The model under review builds one solid part; all positions refer to its coordinate system, in mm. A direction names the side the tool comes from. Coordinates: 2 decimals unless noted, no trailing zeros. Write each loop counter-clockwise with the first axis right and the second up, starting at its lowest first coordinate (ties: lowest second). Pieces come first, ordered by that corner, then holes.
```python
from build123d import *

# Parameters (mm, degrees)
ESBO_O1_W                                            = 105
ESBO_O1_H                                            = 50
RESSALTO_EXTRUS_O1_DEPTH                             = 6.35
FURO_DE_DI_METRO_2_5_2_5_1_D                         = 2.5
FURO_DE_DI_METRO_2_5_2_5_1_DEPTH                     = 6.35
REBAIXO_PARA_PARAFUSO_DE_M_QUINA_DE_CABE_D           = 2.2
REBAIXO_PARA_PARAFUSO_DE_M_QUINA_DE_CABE_DEPTH       = 6.35
REBAIXO_PARA_PARAFUSO_DE_M_QUINA_DE_CABE_CBORE_D     = 4.4
REBAIXO_PARA_PARAFUSO_DE_M_QUINA_DE_CABE_CBORE_DEPTH = 2.25
REBAIXO_PARA_PARAFUSO_DE_M_QUINA_DE_2_D              = 4.3
REBAIXO_PARA_PARAFUSO_DE_M_QUINA_DE_2_CBORE_D        = 8
REBAIXO_PARA_PARAFUSO_DE_M_QUINA_DE_2_CBORE_DEPTH    = 4.25
REBAIXO_PARA_PARAFUSO_DE_M_QUINA_DE_3_D              = 4.3
REBAIXO_PARA_PARAFUSO_DE_M_QUINA_DE_3_DEPTH          = 6.35
REBAIXO_PARA_PARAFUSO_DE_M_QUINA_DE_3_CBORE_D        = 8
REBAIXO_PARA_PARAFUSO_DE_M_QUINA_DE_3_CBORE_DEPTH    = 4.25
FILETE1_R                                            = 3
ESBO_O11_R                                           = 4
RESSALTO_EXTRUS_O2_DEPTH                             = 6.35


with BuildPart() as part:
    # Esboço1 → Ressalto-extrusão1 (new body)
    with BuildSketch(Plane.XY.offset(6.35)):
        with Locations((52.5, 12)):
            Rectangle(ESBO_O1_W, ESBO_O1_H)
    extrude(amount=-RESSALTO_EXTRUS_O1_DEPTH)

    # Furo de diâmetro Ø2.5 (2.5)1
    with Locations(Plane(origin=(0, 0, 0), x_dir=(-1, 0, 0), z_dir=(0, 0, -1))):
        with Locations((-95.5, 17), (-95.5, 7)):
            Hole(FURO_DE_DI_METRO_2_5_2_5_1_D / 2, depth=FURO_DE_DI_METRO_2_5_2_5_1_DEPTH)

    # Rebaixo para parafuso de m_quina de cabe
    with Locations(Plane.XY.offset(6.35)):
        with Locations((45.856, 22), (45.856, 2), (45.856, 12)):
            CounterBoreHole(REBAIXO_PARA_PARAFUSO_DE_M_QUINA_DE_CABE_D / 2, REBAIXO_PARA_PARAFUSO_DE_M_QUINA_DE_CABE_CBORE_D / 2, REBAIXO_PARA_PARAFUSO_DE_M_QUINA_DE_CABE_CBORE_DEPTH, depth=REBAIXO_PARA_PARAFUSO_DE_M_QUINA_DE_CABE_DEPTH)

    # Rebaixo para parafuso de m_quina de  2 (through all)
    with Locations(Plane(origin=(0, 0, 0), x_dir=(-1, 0, 0), z_dir=(0, 0, -1))):
        with Locations((-6, -5.5), (-6, 29.5), (-71, -1.5), (-71, 25.5)):
            CounterBoreHole(REBAIXO_PARA_PARAFUSO_DE_M_QUINA_DE_2_D / 2, REBAIXO_PARA_PARAFUSO_DE_M_QUINA_DE_2_CBORE_D / 2, REBAIXO_PARA_PARAFUSO_DE_M_QUINA_DE_2_CBORE_DEPTH)

    # Rebaixo para parafuso de m_quina de  3
    with Locations(Plane.XY.offset(6.35)):
        with Locations((5, 21), (5, 3), (29, 3), (29, 21), (56, 3), (56, 21), (80, 21), (80, 3)):
            CounterBoreHole(REBAIXO_PARA_PARAFUSO_DE_M_QUINA_DE_3_D / 2, REBAIXO_PARA_PARAFUSO_DE_M_QUINA_DE_3_CBORE_D / 2, REBAIXO_PARA_PARAFUSO_DE_M_QUINA_DE_3_CBORE_DEPTH, depth=REBAIXO_PARA_PARAFUSO_DE_M_QUINA_DE_3_DEPTH)

    # Filete1
    filete1_edges = [part.edges().sort_by_distance(p)[0] for p in [
        (105, 37, 3.175),
        (105, -13, 3.175),
        (0, -13, 3.175),
        (0, 37, 3.175),
    ]]
    fillet(filete1_edges, radius=FILETE1_R)

    # Esboço11 → Ressalto-extrusão2 (add)
    with BuildSketch(Plane(origin=(0, 0, 0), x_dir=(-1, 0, 0), z_dir=(0, 0, -1))):
        with Locations((-71, -1.5)):
            Circle(ESBO_O11_R)
        with Locations((-71, 25.5)):
            Circle(ESBO_O11_R)
    extrude(amount=-RESSALTO_EXTRUS_O2_DEPTH)


solid = part.part
```
Item 1: Take a section at B-B, the plane x = 5. Count the separate pieces of the cut face and the enclosed holes in it, plus the area to 3 significant figures.
Solved:
separate pieces: 5
enclosed holes: 0
area: 150 mm2
Item 2: For pin 1 (2 mm diameter, centred on x = 95.5, y = 7, fed in from -Z); pin 2 (13 mm diameter, centred on x = 29, y = 3, fed in from -Z); pin 3 (5 mm diameter, centred on x = 6, y = -5.5, fed in from -Z); pin 4 (3 mm diameter, centred on x = 45.856, y = 2, fed in from +Z), all flat-tipped, find the tip position at first contact; note any pin that passes through.
Solved:
pin 1: passes through
pin 2: stops at z = 0
pin 3: stops at z = 4.25
pin 4: stops at z = 4.1
Item 3: Machinability: for faces 5 (the face through (4.133, -0.905, 4.255)), 6 (the face through (44.84, 11.58, 2.02)), 7 (the face through (6.521, 33.466, 2.095)), which of the approach directions +Z, -Z, +X, -X, +Y, -Y give a long, thin tool a straight path to every point of the face, cutting with its end or side? Answer none if there is none.
Solved:
face 5: +Z
face 6: +Z, -Z
face 7: -Z
Item 4: Take a section at A-A, the plane x = 56. Write out the cut boundary in (y, z), plus the area to 3 significant figures.
Solved:
outline: (-13, 0) - (0.85, 0) - (0.85, 2.1) - (-1, 2.1) - (-1, 6.35) - (-13, 6.35) - close; (5.15, 0) - (18.85, 0) - (18.85, 2.1) - (17, 2.1) - (17, 6.35) - (7, 6.35) - (7, 2.1) - (5.15, 2.1) - close; (23.15, 0) - (37, 0) - (37, 6.35) - (25, 6.35) - (25, 2.1) - (23.15, 2.1) - close
area: 231 mm2
Item 5: To check wall thickness, follow line 1 along Y through (x, z) = (29, 5.4); line 2 along Y through (x, z) = (80, 0.75); line 3 along Y through (x, z) = (6, 1.45). State the ranges of each line that lie inside material, in increasing order.
Solved:
line 1: y = -13 to -1, 7 to 17, 25 to 37
line 2: y = -13 to 0.85, 5.15 to 18.85, 23.15 to 37
line 3: y = -13 to -9.5, -1.5 to 1.1, 4.9 to 19.1, 22.9 to 25.5, 33.5 to 37
Item 6: Mouldability with a two-part tool opening along X and no side actions: class faces 1 (the face through (104.1, 36.14, 3.13)), 2 (the face through (52, 12, 6.35)), 3 (the face through (82.15, 3.09, 1.04)), 4 (the face through (47.954, 2.661, 5.241)) as pulls with the +X half, pulls with the -X half, needs draft (parallel to the pull), parting line crosses it, or undercut.
Solved:
face 1: pulls with the +X half
face 2: needs draft
face 3: undercut
face 4: undercut
